Can you work these out from the model? Positions are in its coordinate system, mm. A direction names the side the tool comes from. Coordinates: 2 decimals unless noted, no trailing zeros. Order: outer loops, then holes, each group sorted by start corner. A loop starts at its lowest first (then second) coordinate and runs counter-clockwise, first axis right, second up. Notation, with made-up numbers: (66.5, 49.5) -> (70.5, 49.5) arc R34 cw to (70.5, 79.5) -> close; hole circle Ø11 at (32, -20). An arc over 180 degrees is marked (long way). Answer in a Markdown table with one row per item.
```python
from build123d import *

# Parameters (mm, degrees)
SKETCH1_R           = 25
BOSS_EXTRUDE1_DEPTH = 700
CUT_EXTRUDE1_START  = -50
SKETCH2_R           = 25
SKETCH2_R_2         = 13.119240587
CUT_EXTRUDE1_DEPTH  = 50
SKETCH3_R           = 25
SKETCH3_R_2         = 11.320441419
CUT_EXTRUDE2_DEPTH  = 30


with BuildPart() as part:
    # Sketch1 → Boss-Extrude1 (new body)
    with BuildSketch(Plane.XY):
        Circle(SKETCH1_R)
    extrude(amount=BOSS_EXTRUDE1_DEPTH)

    # Sketch2 → Cut-Extrude1 (cut)
    with BuildSketch(Plane.XY.offset(700).offset(CUT_EXTRUDE1_START)):
        Circle(SKETCH2_R)
        Circle(SKETCH2_R_2, mode=Mode.SUBTRACT)
    extrude(amount=CUT_EXTRUDE1_DEPTH, mode=Mode.SUBTRACT)

    # Sketch3 → Cut-Extrude2 (cut)
    with BuildSketch(Plane(origin=(0, 0, 0), x_dir=(-1, 0, 0), z_dir=(0, 0, -1))):
        Circle(SKETCH3_R)
        Circle(SKETCH3_R_2, mode=Mode.SUBTRACT)
    extrude(amount=-CUT_EXTRUDE2_DEPTH, mode=Mode.SUBTRACT)


solid = part.part
```
(1) On a 3-axis mill with a long thin cutter (end or side, diameter ignored), from which of +Z, -Z, +X, -X, +Y, -Y can I reach the whole of each face in a straight line? I mean faces 1 (the flat face through (0, 0, 700)), 2 (the cylindrical face through (-6.086, 9.545, 14.79)), 3 (the cylindrical face through (-2.84, -12.81, 674.65)). Say none if no direction works.
Response values:
| item | result |
|---|---|
| face 1 | +Z, +X, -X, +Y, -Y |
| face 2 | -Z |
| face 3 | +Z |
(2) Suppose I cut it at C-C (z = 203). Please give me the cut outline in (x, y).
Response values:
| item | result |
|---|---|
| outline | circle Ø50 at (0, 0) |
(3) I need wall thicknesses on line 1 (X direction, y = 2, z = 184.5); line 2 (Z direction, x = 17, y = 9.5); line 3 (Z direction, x = -7, y = -10.5). Which ranges of each line are inside material? Lowest first, please. Write a range as [from, to].
Response values:
| item | result |
|---|---|
| line 1 | [-24.92, 24.92] |
| line 2 | [30, 650] |
| line 3 | [30, 700] |
(4) Suppose I cut it at A-A (x = 0). Please give me the cut outline in (y, z), and give its area (3 significant figures).
Response values:
| item | result |
|---|---|
| outline | (-25, 30) -> (-11.32, 30) -> (-11.32, 0) -> (11.32, 0) -> (11.32, 30) -> (25, 30) -> (25, 650) -> (13.12, 650) -> (13.12, 700) -> (-13.12, 700) -> (-13.12, 650) -> (-25, 650) -> close |
| area | 33,000 mm2 |
(5) Will these pins go through, and if not, where does the flat tip stop? pin 1 Ø3 at (x, y) = (9.5, 11.5) entering from +Z; pin 2 Ø2 at (x, z) = (-19.5, 251) entering from +Y; pin 3 Ø3 at (y, z) = (12.5, 84.5) entering from +X.
Response values:
| item | result |
|---|---|
| pin 1 | z = 650 |
| pin 2 | y = 16.82 |
| pin 3 | x = 22.45 |
